The listing builds one solid part. Answer for the finished solid, in the listing's coordinates (mm). A direction names the side the tool comes from. Give positions to 0.01 mm unless a question says otherwise; leave off trailing zeros. Write each loop counter-clockwise with the first axis right and the second up, starting at its lowest first coordinate (ties: lowest second). Pieces come first, ordered by that corner, then holes. Notation, with made-up numbers: (-2, 63.25) -> (20, 63.25) arc R16 ccw to (20, 86.25) -> close; hole circle Ø2 at (1.25, 23.5). An arc over 180 degrees is marked (long way). Put each result on its own line as item: value. Start each with the question number.
1) A cutting plane is placed at D-D (z = 14.5). Write down the section's boundary in (x, y).
2) A cutting plane is placed at C-C (z = -6.5). Write down the section's boundary in (x, y), then the cut area to 3 significant figures.
3) A cutting plane is placed at B-B (x = -1.5). Write down the section's boundary in (y, z), then the cut area to 3 significant figures.
4) For a pull along Y with two mould halves and no side action, classify faces 1 (the flat face through (0, -4.6, 17)), 2 (the flat face through (-25, -1, 16)), 3 (the flat face through (-30, 6.3, -24)) as released by +Y, released by -Y, zero draft, split by the parting line, or undercut.
5) Find the intervals of material crossed by line 1 along X through (y, z) = (2, -26); line 2 along X through (y, z) = (-2, -23); line 3 along Y through (x, z) = (7, 20.5), in increasing order. Write a range as from..to.
6) Flat-ended cylindrical pins translate along their axes: pin 1 Ø1 at (x, y) = (16.5, -2) entering from -Z; pin 2 Ø4 at (y, z) = (-3, 31.5) entering from -X; pin 3 Ø6 at (x, y) = (-11, 0.5) entering from -Z. Find the tip coordinate at first contact, or state that the pin passes through.
7) For faces 4 (the flat face through (28.3, 7, -24)), 5 (the flat face through (28.3, -2, -33)), 6 (the flat face through (-30, 2, 19.3)), 7 (the flat face through (30, 2, 19.3)), 8 (the flat face through (-28.3, -2, 33)), determine the directions among +Z, -Z, +X, -X, +Y, -Y from which every point of the face is accessible in a straight line to the end or side of a thin tool.
from build123d import *

# Parameters (mm, degrees)
STOCK_BATTERY_START                           = -4.6
STOCK_BATTERY_AND_MICRO_COMPARTMENT_1_DEPTH   = 4.6
STOCK_BATTERY_AND_MICRO_COMPARTMENT_1_2_DEPTH = 2.3
BOSS_EXTRUDE1_START                           = -4.6
BOSS_EXTRUDE1_DEPTH                           = 4.6
CUT_EXTRUDE1_DEPTH                            = 2.3
BOSS_EXTRUDE2_DEPTH                           = 0.3
SKETCH4_W                                     = 74
SKETCH4_H                                     = 4.9
BOSS_EXTRUDE3_DEPTH                           = 0.3
BOSS_EXTRUDE4_START                           = -56.3
SKETCH4_2_W                                   = 74
SKETCH4_2_H                                   = 4.9
BOSS_EXTRUDE4_DEPTH                           = 0.3
SKETCH5_W                                     = 10
SKETCH5_H                                     = 12.9
BOSS_EXTRUDE5_DEPTH                           = 3
BOSS_EXTRUDE7_START                           = -56.6
SKETCH5_2_W                                   = 10
SKETCH5_2_H                                   = 12.9
BOSS_EXTRUDE7_DEPTH                           = 3
CUT_EXTRUDE2_DEPTH                            = 81
CUT_EXTRUDE2_DEPTH_BACK                       = 10
CUT_EXTRUDE3_DEPTH                            = 128
CUT_EXTRUDE3_DEPTH_BACK                       = 10
BOSS_EXTRUDE8_REACH                           = 51.27
BOSS_EXTRUDE8_DIRECTION_2_DEPTH               = 0.03
BOSS_EXTRUDE9_DEPTH                           = 2
SPLIT1_START                                  = 0.33
SPLIT1_DEPTH                                  = 2
SPLIT1_START_2                                = -2.3
SPLIT1_2_DEPTH                                = 2.63


# Read off the part's stored shape, not the designer's step: Stock-Battery and Micro compartment-1, Split1
with BuildPart() as part:
    # Stock-Battery and Micro compartment-1 ou → Stock-Battery and Micro compartment-1 (new body)
    with BuildSketch(Plane(origin=(0, 0, 0), x_dir=(1, 0, 0), z_dir=(0, 1, 0)).offset(STOCK_BATTERY_START)):
        with BuildLine():
            Line((-28, 37.2), (-28, -36.8))
            Line((-28, -36.8), (28, -36.8))
            Line((28, -36.8), (28, 37.2))
            Line((28, 37.2), (25, 37.2))
            Line((25, 37.2), (25, 9.8))
            ThreePointArc((25, 9.8), (0, -15.2), (-25, 9.8))
            Line((-25, 9.8), (-25, 37.2))
            Line((-25, 37.2), (-28, 37.2))
        make_face()
    extrude(amount=STOCK_BATTERY_AND_MICRO_COMPARTMENT_1_DEPTH)

    # Stock-Battery and Micro compartment- 2 → Stock-Battery and Micro compartment-1 2 (add)
    with BuildSketch(Plane(origin=(0, 0, 0), x_dir=(1, 0, 0), z_dir=(0, 1, 0)).offset(STOCK_BATTERY_START)):
        with BuildLine():
            Line((-22.7, 37.2), (-25, 37.2))
            Line((-25, 37.2), (-25, 9.8))
            ThreePointArc((-25, 9.8), (0, -15.2), (25, 9.8))
            Line((25, 9.8), (25, 37.2))
            Line((25, 37.2), (22.7, 37.2))
            Line((22.7, 37.2), (22.7, 9.8))
            ThreePointArc((22.7, 9.8), (0, -12.9), (-22.7, 9.8))
            Line((-22.7, 9.8), (-22.7, 37.2))
        make_face()
    extrude(amount=STOCK_BATTERY_AND_MICRO_COMPARTMENT_1_2_DEPTH)

    # Sketch2 → Boss-Extrude1 (add)
    with BuildSketch(Plane(origin=(0, 0, 0), x_dir=(1, 0, 0), z_dir=(0, 1, 0)).offset(BOSS_EXTRUDE1_START)):
        with BuildLine():
            Line((0, -11.2), (-13.564659966, -11.2))
            ThreePointArc((-13.564659966, -11.2), (0, -15.2), (13.564659966, -11.2))
            Line((13.564659966, -11.2), (0, -11.2))
        make_face()
    extrude(amount=BOSS_EXTRUDE1_DEPTH)

    # Sketch1 → Cut-Extrude1 (cut)
    with BuildSketch(Plane(origin=(0, 0, 0), x_dir=(1, 0, 0), z_dir=(0, 1, 0))):
        with BuildLine():
            Line((14.142135624, -13.2), (-14.142135624, -13.2))
            ThreePointArc((-14.142135624, -13.2), (-20.591241985, -7.66427077), (-25, -0.398039027))
            Line((-25, -0.398039027), (-25, -32.8))
            Line((-25, -32.8), (25, -32.8))
            Line((25, -32.8), (25, -0.398039027))
            ThreePointArc((25, -0.398039027), (20.591241985, -7.66427077), (14.142135624, -13.2))
        make_face()
    extrude(amount=-CUT_EXTRUDE1_DEPTH, mode=Mode.SUBTRACT)

    # Sketch3 → Boss-Extrude2 (add)
    with BuildSketch(Plane(origin=(0, 0, 0), x_dir=(1, 0, 0), z_dir=(0, 1, 0))):
        with BuildLine():
            Line((-25, 37.2), (-28, 37.2))
            Line((-28, 37.2), (-28, -36.8))
            Line((-28, -36.8), (28, -36.8))
            Line((28, -36.8), (28, 37.2))
            Line((28, 37.2), (25, 37.2))
            Line((25, 37.2), (25, 9.8))
            ThreePointArc((25, 9.8), (21.955824958, -2.155824958), (13.564659966, -11.2))
            Line((13.564659966, -11.2), (-13.564659966, -11.2))
            ThreePointArc((-13.564659966, -11.2), (-21.955824958, -2.155824958), (-25, 9.8))
            Line((-25, 9.8), (-25, 37.2))
        make_face()
        with BuildLine():
            Line((-25, -32.8), (25, -32.8))
            Line((25, -32.8), (25, -0.398039027))
            ThreePointArc((25, -0.398039027), (20.591241985, -7.66427077), (14.142135624, -13.2))
            Line((14.142135624, -13.2), (-14.142135624, -13.2))
            ThreePointArc((-14.142135624, -13.2), (-20.591241985, -7.66427077), (-25, -0.398039027))
            Line((-25, -0.398039027), (-25, -32.8))
        make_face(mode=Mode.SUBTRACT)
    extrude(amount=BOSS_EXTRUDE2_DEPTH)

    # Sketch4 → Boss-Extrude3 (add)
    with BuildSketch(Plane(origin=(28, 0, 0), x_dir=(0, 0, -1), z_dir=(1, 0, 0))):
        with Locations((0.2, -2.15)):
            Rectangle(SKETCH4_W, SKETCH4_H)
    extrude(amount=BOSS_EXTRUDE3_DEPTH)

    # Sketch4<2> → Boss-Extrude4 (add)
    with BuildSketch(Plane(origin=(28, 0, 0), x_dir=(0, 0, -1), z_dir=(1, 0, 0)).offset(BOSS_EXTRUDE4_START)):
        with Locations((0.2, -2.15)):
            Rectangle(SKETCH4_2_W, SKETCH4_2_H)
    extrude(amount=BOSS_EXTRUDE4_DEPTH)

    # Sketch5 → Boss-Extrude5 (add)
    with BuildSketch(Plane(origin=(28.3, 0, 0), x_dir=(0, 0, -1), z_dir=(1, 0, 0))):
        with Locations((-24.3, 1.85)):
            Rectangle(SKETCH5_W, SKETCH5_H)
        with Locations((24.3, 1.85)):
            Rectangle(SKETCH5_W, SKETCH5_H)
    extrude(amount=BOSS_EXTRUDE5_DEPTH)

    # Sketch5<2> → Boss-Extrude7 (add)
    with BuildSketch(Plane(origin=(28.3, 0, 0), x_dir=(0, 0, -1), z_dir=(1, 0, 0)).offset(BOSS_EXTRUDE7_START)):
        with Locations((-24.3, 1.85)):
            Rectangle(SKETCH5_2_W, SKETCH5_2_H)
        with Locations((24.3, 1.85)):
            Rectangle(SKETCH5_2_W, SKETCH5_2_H)
    extrude(amount=-BOSS_EXTRUDE7_DEPTH)

    # Sketch8 → Cut-Extrude2 (cut, two sides: drawn at the far end of the back side and taken through both)
    with BuildSketch(Plane(origin=(-28.3, 0, 0), x_dir=(0, 0, -1), z_dir=(1, 0, 0)).offset(-CUT_EXTRUDE2_DEPTH_BACK)):
        with BuildLine():
            Line((22.8, 2.3), (25.8, 2.3))
            ThreePointArc((25.8, 2.3), (26.8, 4.3), (25.8, 6.3))
            Line((25.8, 6.3), (22.8, 6.3))
            ThreePointArc((22.8, 6.3), (21.8, 4.3), (22.8, 2.3))
        make_face()
    extrude(amount=CUT_EXTRUDE2_DEPTH + CUT_EXTRUDE2_DEPTH_BACK, mode=Mode.SUBTRACT)

    # Sketch9 → Cut-Extrude3 (cut, two sides: drawn at the far end of the back side and taken through both)
    with BuildSketch(Plane(origin=(-28.3, 0, 0), x_dir=(0, 0, -1), z_dir=(1, 0, 0)).offset(-CUT_EXTRUDE3_DEPTH_BACK)):
        with BuildLine():
            Line((-25.8, 2.3), (-22.8, 2.3))
            ThreePointArc((-22.8, 2.3), (-21.8, 4.3), (-22.8, 6.3))
            Line((-22.8, 6.3), (-25.8, 6.3))
            ThreePointArc((-25.8, 6.3), (-26.8, 4.3), (-25.8, 2.3))
        make_face()
    extrude(amount=CUT_EXTRUDE3_DEPTH + CUT_EXTRUDE3_DEPTH_BACK, mode=Mode.SUBTRACT)


with BuildPart() as body_2:

    # Sketch10 → Boss-Extrude8 (new, up to next)
    with BuildSketch(Plane(origin=(0, 0.3, 0), x_dir=(1, 0, 0), z_dir=(0, 1, 0)), mode=Mode.PRIVATE) as boss_extrude8_sk1:
        with BuildLine():
            Line((14.142135624, -13.2), (-14.142135624, -13.2))
            ThreePointArc((-14.142135624, -13.2), (-20.180507814, -8.137310399), (-24.5, -1.546805718))
            Line((-24.5, -1.546805718), (-24.5, -5.716120649))
            ThreePointArc((-24.5, -5.716120649), (-20.163977484, -11.042600894), (-14.696938457, -15.2))
            Line((-14.696938457, -15.2), (14.696938457, -15.2))
            ThreePointArc((14.696938457, -15.2), (20.163977484, -11.042600894), (24.5, -5.716120649))
            Line((24.5, -5.716120649), (24.5, -1.546805718))
            ThreePointArc((24.5, -1.546805718), (20.180507814, -8.137310399), (14.142135624, -13.2))
        make_face()
    boss_extrude8_tool1 = extrude(boss_extrude8_sk1.sketch, amount=-BOSS_EXTRUDE8_REACH, mode=Mode.PRIVATE) - part.part
    add(boss_extrude8_tool1.solids().sort_by_distance((0, 0.3, 13.708666))[0])

    # Sketch10 → Boss-Extrude8 direction 2 (add)
    with BuildSketch(Plane(origin=(0, 0.3, 0), x_dir=(1, 0, 0), z_dir=(0, 1, 0))):
        with BuildLine():
            Line((14.142135624, -13.2), (-14.142135624, -13.2))
            ThreePointArc((-14.142135624, -13.2), (-20.180507814, -8.137310399), (-24.5, -1.546805718))
            Line((-24.5, -1.546805718), (-24.5, -5.716120649))
            ThreePointArc((-24.5, -5.716120649), (-20.163977484, -11.042600894), (-14.696938457, -15.2))
            Line((-14.696938457, -15.2), (14.696938457, -15.2))
            ThreePointArc((14.696938457, -15.2), (20.163977484, -11.042600894), (24.5, -5.716120649))
            Line((24.5, -5.716120649), (24.5, -1.546805718))
            ThreePointArc((24.5, -1.546805718), (20.180507814, -8.137310399), (14.142135624, -13.2))
        make_face()
    extrude(amount=BOSS_EXTRUDE8_DIRECTION_2_DEPTH)

    # Sketch11 → Boss-Extrude9 (add)
    with BuildSketch(Plane(origin=(0, 0.33, 0), x_dir=(1, 0, 0), z_dir=(0, 1, 0))):
        with BuildLine():
            Line((-24.5, 8.453194282), (-24.5, -5.716120649))
            ThreePointArc((-24.5, -5.716120649), (-20.163977484, -11.042600894), (-14.696938457, -15.2))
            Line((-14.696938457, -15.2), (14.696938457, -15.2))
            ThreePointArc((14.696938457, -15.2), (20.163977484, -11.042600894), (24.5, -5.716120649))
            Line((24.5, -5.716120649), (24.5, -1.546805718))
            Line((24.5, -1.546805718), (24.5, 8.453194282))
            Line((24.5, 8.453194282), (-24.5, 8.453194282))
        make_face()
    extrude(amount=BOSS_EXTRUDE9_DEPTH)

    # Split1 outline → Split1 (cut)
    with BuildSketch(Plane(origin=(0, 0, 0), x_dir=(1, 0, 0), z_dir=(0, 1, 0)).offset(SPLIT1_START)):
        with BuildLine():
            Line((24.5, -5.716120649), (24.5, 8.453194282))
            Line((24.5, 8.453194282), (-24.5, 8.453194282))
            Line((-24.5, 8.453194282), (-24.5, -5.716120649))
            ThreePointArc((-24.5, -5.716120649), (-20.163977484, -11.042600894), (-14.696938457, -15.2))
            Line((-14.696938457, -15.2), (14.696938457, -15.2))
            ThreePointArc((14.696938457, -15.2), (20.163977484, -11.042600894), (24.5, -5.716120649))
        make_face()
    extrude(amount=SPLIT1_DEPTH, mode=Mode.SUBTRACT)

    # Split1 2 outline → Split1 2 (cut)
    with BuildSketch(Plane(origin=(0, 0, 0), x_dir=(1, 0, 0), z_dir=(0, 1, 0)).offset(SPLIT1_START_2)):
        with BuildLine():
            Line((24.5, -5.716120649), (24.5, -1.546805718))
            ThreePointArc((24.5, -1.546805718), (20.180507814, -8.137310399), (14.142135624, -13.2))
            Line((14.142135624, -13.2), (-14.142135624, -13.2))
            ThreePointArc((-14.142135624, -13.2), (-20.180507814, -8.137310399), (-24.5, -1.546805718))
            Line((-24.5, -1.546805718), (-24.5, -5.716120649))
            ThreePointArc((-24.5, -5.716120649), (-20.163977484, -11.042600894), (-14.696938457, -15.2))
            Line((-14.696938457, -15.2), (14.696938457, -15.2))
            ThreePointArc((14.696938457, -15.2), (20.163977484, -11.042600894), (24.5, -5.716120649))
        make_face()
    extrude(amount=SPLIT1_2_DEPTH, mode=Mode.SUBTRACT)


solid = part.part
Reply:
1. outline: (-28.3, -4.6) -> (28.3, -4.6) -> (28.3, 0.3) -> (25, 0.3) -> (25, -2.3) -> (-25, -2.3) -> (-25, 0.3) -> (-28.3, 0.3) -> close
2. outline: (-28.3, -4.6) -> (-22.46, -4.6) -> (-22.46, -2.3) -> (-24.78, -2.3) -> (-24.78, 0.3) -> (-28.3, 0.3) -> close; (22.46, -4.6) -> (28.3, -4.6) -> (28.3, 0.3) -> (24.78, 0.3) -> (24.78, -2.3) -> (22.46, -2.3) -> close
2. area: 45.2 mm2
3. outline: (-4.6, 11.2) -> (0.3, 11.2) -> (0.3, 13.2) -> (-2.3, 13.2) -> (-2.3, 32.8) -> (0.3, 32.8) -> (0.3, 36.8) -> (-4.6, 36.8) -> close
3. area: 74.5 mm2
4. face 1: released by -Y
4. face 2: zero draft
4. face 3: undercut
5. line 1: x = -31.3..-28.3, 28.3..31.3
5. line 2: x = -31.3..-25, 25..31.3
5. line 3: y = -4.6..-2.3
6. pin 1: stops at z = 5.36
6. pin 2: stops at x = -28.3
6. pin 3: stops at z = 9.42
7. face 4: +Z, -Z, +Y
7. face 5: -Z, +X, +Y, -Y
7. face 6: -X, +Y, -Y
7. face 7: +X, +Y, -Y
7. face 8: +Z, -X, +Y, -Y
